Part model, mm, in its own coordinate system. A direction names the side the tool comes from. Round coordinates to 2 decimals unless told otherwise and drop trailing zeros. Loops run counter-clockwise (first coordinate to the right, second up) from the corner with the lowest first, then second, coordinate; pieces in that order, holes last. Notation, with made-up numbers: M 2,55.25 L 41,55.25 A31 cw 41,80.25 Z; hole C 74,-25 d5. An arc over 180 degrees is marked long. Put each result on its own line as item: value. Start each with the question number.
1) Drop flat-ended pins along their axis: pin 1 Ø0.8 at (x, y) = (14.5, 2.5) entering from +Z; pin 2 Ø3.5 at (x, z) = (22, 5) entering from -Y; pin 3 Ø1 at (y, z) = (0.5, -1) entering from +X; pin 4 Ø2 at (x, z) = (9, 2.5) entering from +Y. Give the stop position or say it passes through.
2) Which spindle directions (+Z, -Z, +X, -X, +Y, -Y) get a long thin tool onto all of the face, cutting with end or side? Do faces 4 (the cylindrical face through (19.57, -1.99, -0.05)), 5 (the flat face through (14.465, -2.26, 1.253)), 6 (the flat face through (12.6, 2, 2.1)), 7 (the cylindrical face through (12.43, -1.99, 5.05)). Say none if no direction does.
3) Slice it at A-A on y = 1.25. Give the cut face in (x, z).
4) Slice it at B-B on z = 2. Give the cut face in (x, y), then the cut area to 3 significant figures.
5) Pull direction Z, two halves, no side cores. Call faces 1 (the flat face through (9.39, 2.51, 3.88)), 2 (the flat face through (20, -2, 3)), 3 (the flat face through (16.3, 1.9, 7.4)): +Z half, -Z half, draft (parallel to the pull), parting line (faces both ways), or undercut.
6) Probe line 1 along X through (y, z) = (2.75, 2.75); line 2 along X through (y, z) = (2.5, 3.75); line 3 along X through (y, z) = (-2.5, 3.25). List the from-to ranges inside material, lowest first.
```python
from build123d import *

# Parameters (mm, degrees)
BOSS_EXTRUDE1_DEPTH = 3
CHAMFER1_SIZE       = 2.2
BOSS_EXTRUDE2_DEPTH = 3
CUT_EXTRUDE1_DEPTH  = 1
CUT_EXTRUDE2_DEPTH  = 5
FILLET1_R           = 1


with BuildPart() as part:
    # Sketch1 → Boss-Extrude1 (new body)
    with BuildSketch(Plane(origin=(0, 0, 0), x_dir=(1, 0, 0), z_dir=(0, 1, 0))):
        with BuildLine():
            Line((24, -8.5), (33, -8.5))
            ThreePointArc((33, -8.5), (35.474873734, -7.474873734), (36.5, -5))
            Line((36.5, -5), (36.5, 0))
            ThreePointArc((36.5, 0), (35.474873734, 2.474873734), (33, 3.5))
            Line((33, 3.5), (24, 3.5))
            Line((24, 3.5), (0, 3.5))
            ThreePointArc((0, 3.5), (-2.474873734, 2.474873734), (-3.5, 0))
            Line((-3.5, 0), (-3.5, -5))
            ThreePointArc((-3.5, -5), (-2.474873734, -7.474873734), (0, -8.5))
            Line((0, -8.5), (24, -8.5))
        make_face()
    extrude(amount=BOSS_EXTRUDE1_DEPTH)

    # Chamfer1
    chamfer1_edges = [part.edges().sort_by_distance(p)[0] for p in [
        (-3.5, 3, 2.5),
        (-2.474873734, 3, 7.474873734),
        (16.5, 3, 8.5),
        (35.474873734, 3, 7.474873734),
        (36.5, 3, 2.5),
        (35.474873734, 3, -2.474873734),
        (16.5, 3, -3.5),
        (-2.474873734, 3, -2.474873734),
    ]]
    chamfer(chamfer1_edges, length=CHAMFER1_SIZE)

    # Sketch2 → Boss-Extrude2 (add)
    with BuildSketch(Plane.XZ):
        with BuildLine():
            Line((13.5, 5.5), (18.5, 5.5))
            ThreePointArc((18.5, 5.5), (19.560660172, 5.060660172), (20, 4))
            Line((20, 4), (20, 1))
            ThreePointArc((20, 1), (19.560660172, -0.060660172), (18.5, -0.5))
            Line((18.5, -0.5), (13.5, -0.5))
            ThreePointArc((13.5, -0.5), (12.439339828, -0.060660172), (12, 1))
            Line((12, 1), (12, 4))
            ThreePointArc((12, 4), (12.439339828, 5.060660172), (13.5, 5.5))
        make_face()
    extrude(amount=BOSS_EXTRUDE2_DEPTH)

    # Sketch3 → Cut-Extrude1 (cut)
    with BuildSketch(Plane(origin=(0, 3, 0), x_dir=(1, 0, 0), z_dir=(0, 1, 0))):
        Polygon((6.225775105, 0.3), (4.811561543, 0.3), (2.011561543, -2.5), (4.811561543, -5.3), (6.225775105, -5.3), (3.425775105, -2.5), align=None)
        Polygon((9.225775105, 0.3), (7.811561543, 0.3), (5.011561543, -2.5), (7.811561543, -5.3), (9.225775105, -5.3), (6.425775105, -2.5), align=None)
        Polygon((12.225775105, 0.3), (10.811561543, 0.3), (8.011561543, -2.5), (10.811561543, -5.3), (12.225775105, -5.3), (9.425775105, -2.5), align=None)
        Polygon((15.225775105, 0.3), (13.811561543, 0.3), (11.011561543, -2.5), (13.811561543, -5.3), (15.225775105, -5.3), (12.425775105, -2.5), align=None)
    extrude(amount=-CUT_EXTRUDE1_DEPTH, mode=Mode.SUBTRACT)

    # Sketch4 → Cut-Extrude2 (cut)
    with BuildSketch(Plane.ZY.offset(-12)):
        Polygon((1.5, -3), (1, -1.5), (1, 0), (4, 0), (4, -1.5), (3.5, -3), align=None)
    extrude(amount=-CUT_EXTRUDE2_DEPTH, mode=Mode.SUBTRACT)

    # Fillet1
    fillet1_edges = [part.edges().sort_by_distance(p)[0] for p in [
        (12.439339828, 0, 5.060660172),
        (12.439339828, 0, -0.060660172),
        (16, 0, -0.5),
        (19.560660172, 0, -0.060660172),
        (20, 0, 2.5),
        (19.560660172, 0, 5.060660172),
        (16, 0, 5.5),
    ]]
    fillet(fillet1_edges, radius=FILLET1_R)


solid = part.part
```
Recorded:
1. pin 1: stops at z = 7.2
1. pin 2: stops at y = -0.21
1. pin 3: stops at x = 36.46
1. pin 4: stops at y = 3
2. face 4: -Z, +X, -Y
2. face 5: -X
2. face 6: +Y
2. face 7: +Z, -X, -Y
3. outline: M -3.05,0 A3.05 ccw 0,-3.05 L 33,-3.05 A3.05 ccw 36.05,0 L 36.05,5 A3.05 ccw 33,8.05 L 0,8.05 A3.05 ccw -3.05,5 Z
4. outline: M -3.5,0 L 17,0 L 17,-3 L 20,-3 L 20,-1 A1 cw 21,0 L 36.5,0 L 36.5,0.8 L 34.3,3 L 12.93,3 L 12.93,2 L 11.51,2 L 11.51,3 L 9.93,3 L 9.93,2 L 8.51,2 L 8.51,3 L 6.93,3 L 6.93,2 L 5.51,2 L 5.51,3 L 3.93,3 L 3.93,2 L 2.51,2 L 2.51,3 L -1.3,3 L -3.5,0.8 Z
4. area: 119 mm2
5. face 1: undercut
5. face 2: draft
5. face 3: +Z half
6. line 1: x = -1.55 to 2.26, 3.68 to 5.26, 6.68 to 8.26, 9.68 to 11.26, 12.68 to 34.55
6. line 2: x = -1.8 to 3.26, 4.68 to 6.26, 7.68 to 9.26, 10.68 to 12.26, 13.68 to 34.8
6. line 3: x = 17 to 20
